```python
from build123d import *

# Parameters (mm, degrees)
SKETCH1_R           = 75
BOSS_EXTRUDE1_DEPTH = 3
SKETCH2_W           = 15
SKETCH2_H           = 50
D_N_B_NG_D_NH_DEPTH = 1
SKETCH3_R           = 37.559343171
SKETCH3_R_2         = 25
G_N_V_NG_BI_DEPTH   = 20


with BuildPart() as part:
    # Sketch1 → Boss-Extrude1 (new body)
    with BuildSketch(Plane(origin=(0, 0, 0), x_dir=(1, 0, 0), z_dir=(0, 1, 0))):
        with Locations(Location((0, 0, 0), (0, 0, 270))):
            Circle(SKETCH1_R)
    extrude(amount=BOSS_EXTRUDE1_DEPTH)

    # Sketch2 → Dán Băng dính (cut)
    with BuildSketch(Plane.XZ):
        with Locations((-40, 0)):
            Rectangle(SKETCH2_W, SKETCH2_H)
        with Locations((40, 0)):
            Rectangle(SKETCH2_W, SKETCH2_H)
    extrude(amount=-D_N_B_NG_D_NH_DEPTH, mode=Mode.SUBTRACT)

    # Sketch3 → gắn vòng bi (add)
    with BuildSketch(Plane(origin=(0, 3, 0), x_dir=(1, 0, 0), z_dir=(0, 1, 0))):
        with Locations(Location((0, 0, 0), (0, 0, 270))):
            Circle(SKETCH3_R)
        with Locations(Location((0, 0, 0), (0, 0, 270))):
            Circle(SKETCH3_R_2, mode=Mode.SUBTRACT)
    extrude(amount=G_N_V_NG_BI_DEPTH)


solid = part.part
```
CAD build for the part. Positions are in the model's coordinates, mm. A direction names the side the tool comes from. Give positions to 0.01 mm unless a question says otherwise; leave off trailing zeros. Write each loop counter-clockwise with the first axis right and the second up, starting at its lowest first coordinate (ties: lowest second). Pieces come first, ordered by that corner, then holes. Notation, with made-up numbers: (-29, -32) -> (-6, -32) arc R32 cw to (-6, 2) -> close; hole circle Ø2 at (50, 27). An arc over 180 degrees is marked (long way). Write each question's results on one line, items separated by ' | '.
1. Two-plate mould, pull along X, no slides. Class faces 1 (the cylindrical face through (7.509, 12.86, 23.846)), 2 (the flat face through (1, 0, -1)), 3 (the cylindrical face through (-45.636, 1.479, -59.517)), 4 (the flat face through (0, 3, 0)): pulls with the +X half, pulls with the -X half, needs draft (parallel to the pull), parting line crosses it, or undercut.
Geometry check:
face 1: undercut | face 2: needs draft | face 3: parting line crosses it | face 4: undercut
2. Cut at D-D, the plane x = 30. Write the cut outline in (y, z), then the cut area to 3 significant figures.
Geometry check:
outline: (0, -68.74) -> (3, -68.74) -> (3, -22.6) -> (23, -22.6) -> (23, 22.6) -> (3, 22.6) -> (3, 68.74) -> (0, 68.74) -> close | area: 1,320 mm²
3. Cut at B-B, the plane x = 0. Write the cut outline in (y, z).
Geometry check:
outline: (0, -75) -> (3, -75) -> (3, -37.56) -> (23, -37.56) -> (23, -25) -> (3, -25) -> (3, 25) -> (23, 25) -> (23, 37.56) -> (3, 37.56) -> (3, 75) -> (0, 75) -> close
4. Drop flat-ended pins along their axis: P1, Ø0.5, axis at y = 0.5, z = 0, coming from the +X side; P2, Ø10, axis at x = 26, y = 2.5, coming from the +Z side; P3, Ø6, axis at y = 2.5, z = 6.5, coming from the -X side. Give the stop position or say it passes through.
Geometry check:
P1: x = 75 | P2: z = 72 | P3: x = -74.92
5. Cut at A-A, the plane z = 0. Write the cut outline in (x, y).
Geometry check:
outline: (-75, 0) -> (-47.5, 0) -> (-47.5, 1) -> (-32.5, 1) -> (-32.5, 0) -> (32.5, 0) -> (32.5, 1) -> (47.5, 1) -> (47.5, 0) -> (75, 0) -> (75, 3) -> (37.56, 3) -> (37.56, 23) -> (25, 23) -> (25, 3) -> (-25, 3) -> (-25, 23) -> (-37.56, 23) -> (-37.56, 3) -> (-75, 3) -> close
6. Wall check: probe 1 along X at (y, z) = (9.5, 0); probe 2 along X at (y, z) = (22.25, 5); probe 3 along Z at (x, y) = (-14.5, 6.5). Give the ranges that are in metal, low to high. Write a range as [from, to].
Geometry check:
probe 1: [-37.56, -25], [25, 37.56] | probe 2: [-37.23, -24.49], [24.49, 37.23] | probe 3: [-34.65, -20.37], [20.37, 34.65]
7. Which spindle directions (+Z, -Z, +X, -X, +Y, -Y) get a long thin tool onto all of the face, cutting with end or side? Do faces 5 (the flat face through (-15.6, 3, -34.4)), 6 (the flat face through (-25, 23, 8)), 7 (the flat face through (40, 1, 0)). Say none if no direction does.
Geometry check:
face 5: +Y | face 6: +Z, -Z, +X, -X, +Y | face 7: -Y
8. Cut at C-C, the plane y = 18.25. Write the cut outline in (x, z).
Geometry check:
outline: circle Ø75.12 at (0, 0); hole circle Ø50 at (0, 0)
